Input: dimensioned drawing with shaded views. Units: mm. Origin: part minimum x, y, z. A direction names the side the tool comes from. Round coordinates to 2 decimals unless told otherwise and drop trailing zeros. Order: outer loops, then holes, each group sorted by start corner. A loop starts at its lowest first (then second) coordinate and runs counter-clockwise, first axis right, second up. Notation, with made-up numbers: (38, 46.5) - (73, 46.5) arc R21 ccw to (73, 75.5) - close; hole circle Ø6 at (23, 25). An arc over 180 degrees is marked (long way). Put each result on its own line as item: value. Start each with the question number.
(1) Access query for the marked faces 4 and 5. Directions: +Z, -Z, +X, -X, +Y, -Y. A direction counts if a zero-diameter tool reaches every point of the face in a straight line with its end or side. Return the directions, or none.
(2) Material intervals for L1, parallel to X at y = 29, z = 33; L2, parallel to X at y = 16.5, z = 12.5; L3, parallel to Z at x = 13.5, y = 15.5, sorted ascending. Write a range as [from, to].
(3) Section B-B (y = 15). Output: boundary loops of the cut face in (x, z), and give its area (3 significant figures).
(4) Pin query (flat end, axial travel): P1, Ø12, axis at y = 26, z = 5, coming from the -X side; P2, Ø5, axis at x = 18, y = 8.5, coming from the -Z side; P3, Ø2, axis at x = 17, z = 11, coming from the +Y side; P4, Ø7.5, axis at x = 24.5, y = 21, coming from the +Z side. Return the tip coordinate at first contact, or that it passes through.
(5) Section A-A (z = 28). Output: boundary loops of the cut face in (x, y).
(6) Section C-C (z = 4). Output: boundary loops of the cut face in (x, y), and give its area (3 significant figures).
(7) Section D-D (x = 22.5). Output: boundary loops of the cut face in (y, z), and give its area (3 significant figures).
(8) Pull-direction query (X, two-part tool) for the marked faces 1, 2 and 3; classes: released by +X, released by -X, zero draft, split by the parting line, or undercut.
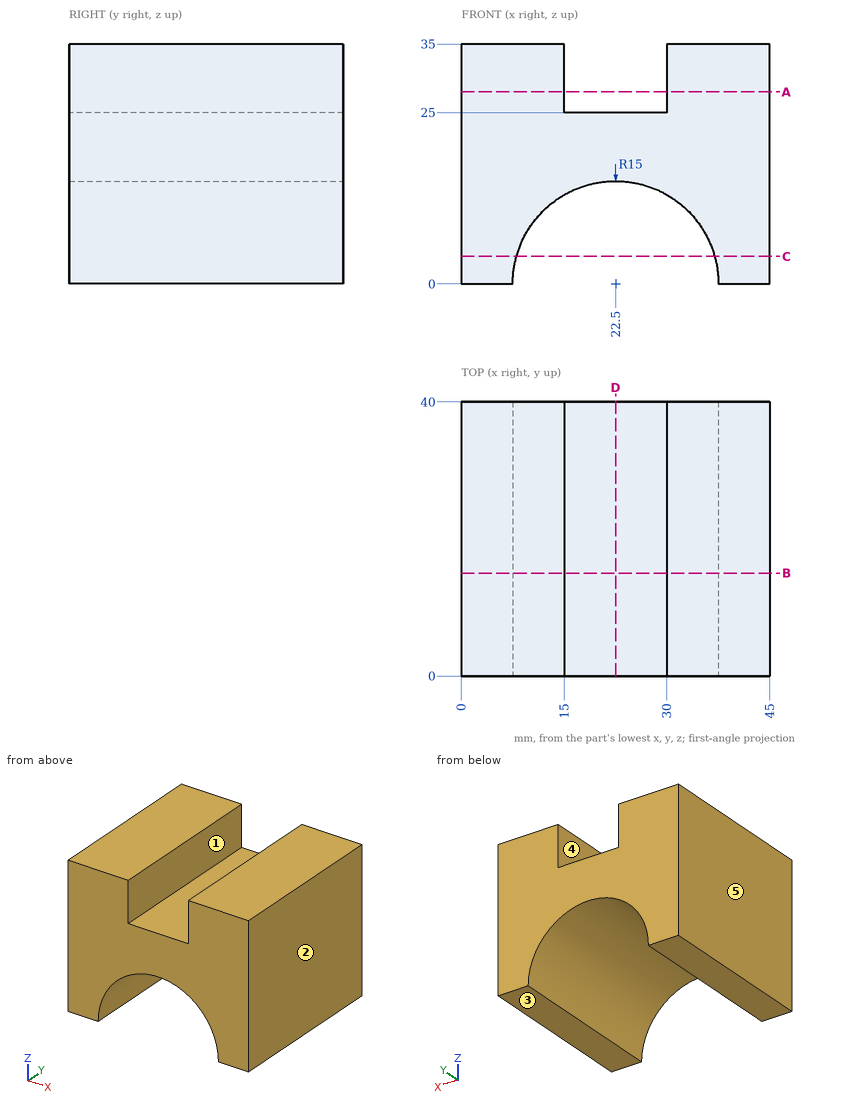
Checks:
1. face 4: +Z, +Y, -Y
1. face 5: +Z, -Z, -X, +Y, -Y
2. L1: x = [0, 15], [30, 45]
2. L2: x = [0, 14.21], [30.79, 45]
2. L3: z = [12, 35]
3. outline: (0, 0) - (7.5, 0) arc R15 cw to (37.5, 0) - (45, 0) - (45, 35) - (30, 35) - (30, 25) - (15, 25) - (15, 35) - (0, 35) - close
3. area: 1,070 mm²
4. P1: stops at x = 0
4. P2: stops at z = 13.27
4. P3: passes through
4. P4: stops at z = 25
5. outline: (0, 0) - (15, 0) - (15, 40) - (0, 40) - close; (30, 0) - (45, 0) - (45, 40) - (30, 40) - close
6. outline: (0, 0) - (8.04, 0) - (8.04, 40) - (0, 40) - close; (36.96, 0) - (45, 0) - (45, 40) - (36.96, 40) - close
6. area: 643 mm²
7. outline: (0, 15) - (40, 15) - (40, 25) - (0, 25) - close
7. area: 400 mm²
8. face 1: undercut
8. face 2: released by +X
8. face 3: zero draft
